Model file for the job. Use its own axes, mm. A direction names the side the tool comes from. Round coordinates to 2 decimals unless told otherwise and drop trailing zeros. Loops run counter-clockwise (first coordinate to the right, second up) from the corner with the lowest first, then second, coordinate; pieces in that order, holes last. Notation, with made-up numbers: (70.25, 9) -> (98.25, 9) arc R12 ccw to (98.25, 16) -> close; hole circle Ø2 at (-26, 66.25). An arc over 180 degrees is marked (long way). Use a Markdown table: item, result.
from build123d import *

# Parameters (mm, degrees)
SKETCH1_W           = 22.225
SKETCH1_H           = 22.225
BOSS_EXTRUDE1_DEPTH = 44.45
CHAMFER1_SIZE       = 3.81
SKETCH2_W           = 25.4
SKETCH2_H           = 25.4
BOSS_EXTRUDE2_DEPTH = 44.45
SKETCH3_W           = 25.4
SKETCH3_H           = 12.7
CUT_EXTRUDE1_DEPTH  = 31.75
SKETCH4_R           = 3.175
CUT_EXTRUDE2_DEPTH  = 94.3255592
SKETCH5_R           = 3.175
CUT_EXTRUDE3_DEPTH  = 22.225


with BuildPart() as part:
    # Sketch1 → Boss-Extrude1 (new body)
    with BuildSketch(Plane.XY):
        Rectangle(SKETCH1_W, SKETCH1_H)
    extrude(amount=BOSS_EXTRUDE1_DEPTH)

    # Chamfer1
    chamfer1_edges = [part.edges().sort_by_distance(p)[0] for p in [
        (11.1125, -11.1125, 22.225),
        (-11.1125, -11.1125, 22.225),
        (-11.1125, 11.1125, 22.225),
        (11.1125, 11.1125, 22.225),
    ]]
    chamfer(chamfer1_edges, length=CHAMFER1_SIZE)

    # Sketch2 → Boss-Extrude2 (add)
    with BuildSketch(Plane.XY.offset(44.45)):
        Rectangle(SKETCH2_W, SKETCH2_H)
    extrude(amount=BOSS_EXTRUDE2_DEPTH)

    # Sketch3 → Cut-Extrude1 (cut)
    with BuildSketch(Plane.XY.offset(88.9)):
        Rectangle(SKETCH3_W, SKETCH3_H)
    extrude(amount=-CUT_EXTRUDE1_DEPTH, mode=Mode.SUBTRACT)

    # Sketch4 → Cut-Extrude2 (cut, through all)
    with BuildSketch(Plane(origin=(0, 12.7, 0), x_dir=(1, 0, 0), z_dir=(0, 1, 0))):
        with Locations(Location((0, -76.2, 0), (0, 0, 270))):
            Circle(SKETCH4_R)
        with BuildLine():
            Line((-12.7, -76.2), (-12.7, -95.25))
            Line((-12.7, -95.25), (12.7, -95.25))
            Line((12.7, -95.25), (12.7, -76.2))
            ThreePointArc((12.7, -76.2), (0, -88.9), (-12.7, -76.2))
        make_face()
    extrude(amount=-CUT_EXTRUDE2_DEPTH, mode=Mode.SUBTRACT)

    # Sketch5 → Cut-Extrude3 (cut)
    with BuildSketch(Plane(origin=(0, 11.1125, 0), x_dir=(1, 0, 0), z_dir=(0, 1, 0))):
        with Locations(Location((0, -31.75, 0), (0, 0, 270))):
            Circle(SKETCH5_R)
        with Locations(Location((0, -15.875, 0), (0, 0, 270))):
            Circle(SKETCH5_R)
    extrude(amount=-CUT_EXTRUDE3_DEPTH, mode=Mode.SUBTRACT)


solid = part.part
Q1. Drill centre lines: L1, parallel to X at y = 5.5, z = 31.75 (1 decimal); L2, parallel to X at y = 11.75, z = 76.2 (3 decimals); L3, parallel to Y at x = -9.25, z = 74. Where is each one in solid material? Low to high. Write a range as from..to.
Results list:
| item | result |
|---|---|
| L1 | x = -11.1..-3.2, 3.2..11.1 |
| L2 | x = -12.7..-3.175, 3.175..12.7 |
| L3 | y = -12.7..-6.35, 6.35..12.7 |
Q2. Band-saw the part on A-A, the plane x = 0. Give the number of separate pieces and of enclosed holes in the cut face, plus the area to 3 significant figures.
Results list:
| item | result |
|---|---|
| separate pieces | 5 |
| enclosed holes | 0 |
| area | 1,350 mm² |
Q3. Band-saw the part on B-B, the plane z = 62.5. Give the cut face in (x, y), plus the area to 3 significant figures.
Results list:
| item | result |
|---|---|
| outline | (-12.7, -12.7) -> (12.7, -12.7) -> (12.7, -6.35) -> (-12.7, -6.35) -> close; (-12.7, 6.35) -> (12.7, 6.35) -> (12.7, 12.7) -> (-12.7, 12.7) -> close |
| area | 323 mm² |
Q4. Flat gauge pins, fed straight in: pin 1 (4 mm diameter, centred on x = 8, y = 2.5, fed in from +Z); pin 2 (7.5 mm diameter, centred on y = 1.5, z = 31.5, fed in from -X); pin 3 (6 mm diameter, centred on x = 2, y = 4.5, fed in from -Z); pin 4 (5 mm diameter, centred on x = 0, z = 76.2, fed in from -Y). Where does each tip first touch, or does it go through?
Results list:
| item | result |
|---|---|
| pin 1 | stops at z = 57.15 |
| pin 2 | stops at x = -11.11 |
| pin 3 | stops at z = 0 |
| pin 4 | passes through |
Q5. Pull direction Y, two halves, no side cores. Call faces 6 (the face through (0, 6.35, 70)), 7 (the face through (12.7, 0, 57)), 8 (the face through (0, 12.7, 66)): released by +Y, released by -Y, zero draft, split by the parting line, or undercut.
Results list:
| item | result |
|---|---|
| face 6 | undercut |
| face 7 | zero draft |
| face 8 | released by +Y |
Q6. Tool access for faces 1 (the face through (-9.181, -9.234, 21.914)), 2 (the face through (0, 11.112, 22)), 3 (the face through (0, -11.112, 22)), 4 (the face through (-11.112, 0, 22)), 5 (the face through (11.112, 0, 22)): list every direction of +Z, -Z, +X, -X, +Y, -Y with a clear straight run to the whole face (end or side of a thin tool).
Results list:
| item | result |
|---|---|
| face 1 | -Z, -X, -Y |
| face 2 | -Z, +X, -X, +Y |
| face 3 | -Z, +X, -X, -Y |
| face 4 | -Z, -X, +Y, -Y |
| face 5 | -Z, +X, +Y, -Y |
Q7. Band-saw the part on D-D, the plane z = 22. Give the cut face in (x, y), plus the area to 3 significant figures.
Results list:
| item | result |
|---|---|
| outline | (-11.11, -7.3) -> (-7.3, -11.11) -> (7.3, -11.11) -> (11.11, -7.3) -> (11.11, 7.3) -> (7.3, 11.11) -> (-7.3, 11.11) -> (-11.11, 7.3) -> close |
| area | 465 mm² |
